```python
from build123d import *

# Parameters (mm, degrees)
BOSS_EXTRU_1_DEPTH      = 40
BOSS_EXTRU_1_DEPTH_BACK = 40
CHANFREIN1_SIZE         = 1.5


with BuildPart() as part:
    # Esquisse1 → Boss.-Extru.1 (new body, two sides)
    with BuildSketch(Plane(origin=(0, 0, 0), x_dir=(0, 0, -1), z_dir=(1, 0, 0))) as boss_extru_1_sk:
        Polygon((-4, 0), (4, 0), (4, -2), (2.5, -3.5), (-2.5, -3.5), (-4, -2), align=None)
    extrude(amount=BOSS_EXTRU_1_DEPTH)
    extrude(boss_extru_1_sk.sketch, amount=-BOSS_EXTRU_1_DEPTH_BACK)

    # Chanfrein1
    chanfrein1_edges = [part.edges().sort_by_distance(p)[0] for p in [
        (40, -3.5, 0),
        (-40, -3.5, 0),
    ]]
    chamfer(chanfrein1_edges, length=CHANFREIN1_SIZE)


solid = part.part
```
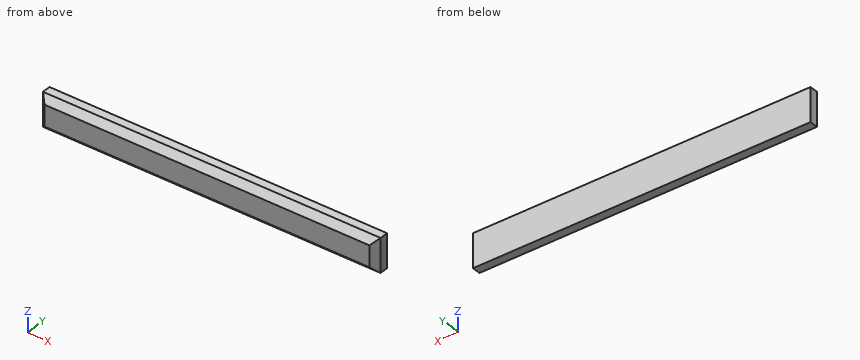
Verification items for the finished model (mm, model axes). Coordinates: 2 decimals unless noted, no trailing zeros. Loops run counter-clockwise (first coordinate to the right, second up) from the corner with the lowest first, then second, coordinate; pieces in that order, holes last. Notation, with made-up numbers: (19.25, 47) -> (38.25, 47) arc R20 cw to (38.25, 68) -> close; hole circle Ø3 at (37.25, -3.75). An arc over 180 degrees is marked (long way). Answer in a Markdown table with one row per item. Add a question column.
1. Depth check by flat-ended pin: P1, Ø3, axis at x = 24.5, z = 3, coming from the +Y side. Enter the tip coordinate at first touch or a pass-through.
2. Section check A-A, the plane x = -2.5. Enter the section's corners in (y, z), then the cut area to 4 significant figures.
3. Material ranges on probe 1 along Y at (x, z) = (-16, 3.5); probe 2 along Y at (x, z) = (-9, 3); probe 3 along Z at (x, y) = (-7, -2.85), recorded low to high. Write a range as [from, to].
4. Section check B-B, the plane y = -2.65. Enter the section's corners in (x, z), then the cut area to 3 significant figures.
Derived:
| question | item | result |
|---|---|---|
| 1 | P1 | stops at y = 0 |
| 2 | outline | (-3.5, -2.5) -> (-2, -4) -> (0, -4) -> (0, 4) -> (-2, 4) -> (-3.5, 2.5) -> close |
| 2 | area | 25.75 mm² |
| 3 | probe 1 | y = [-2.5, 0] |
| 3 | probe 2 | y = [-3, 0] |
| 3 | probe 3 | z = [-3.15, 3.15] |
| 4 | outline | (-39.35, -3.35) -> (39.35, -3.35) -> (39.35, 3.35) -> (-39.35, 3.35) -> close |
| 4 | area | 527 mm² |
